Design review of the part built by this model. Coordinates are the model's own, in mm. Coordinates: 2 decimals unless noted, no trailing zeros. Order: outer loops, then holes, each group sorted by start corner. A loop starts at its lowest first (then second) coordinate and runs counter-clockwise, first axis right, second up. Notation, with made-up numbers: (48, 45) -> (87, 45) arc R26 ccw to (87, 74) -> close; hole circle Ø11 at (-32, 50). An arc over 180 degrees is marked (long way). Write item = value, one per line.
```python
from build123d import *

# Parameters (mm, degrees)
F0_W     = 58.954738
F0_H     = 37.899476
F1_DEPTH = 25.4
F2_R     = 5.08
F3_SIZE  = 5.08


with BuildPart() as f1:
    # F0 (on Front) → F1 (new body)
    with BuildSketch(Plane.XZ):
        Rectangle(F0_W, F0_H)
    extrude(amount=F1_DEPTH)

    # F2
    f2_edges = [f1.edges().sort_by_distance(p)[0] for p in [
        (0, -25.4, 18.949738),
        (0, -25.4, -18.949738),
    ]]
    fillet(f2_edges, radius=F2_R)

    # F3
    f3_edges = [f1.edges().sort_by_distance(p)[0] for p in [
        (0, 0, -18.949738),
        (0, 0, 18.949738),
    ]]
    chamfer(f3_edges, length=F3_SIZE)


solid = f1.part
```
(1) We need section C-C (y = -23). Write out the cut boundary in (x, z).
Report:
outline = (-29.48, -18.19) -> (29.48, -18.19) -> (29.48, 18.19) -> (-29.48, 18.19) -> close
(2) For L1, parallel to Z at x = -11.5, y = -3; L2, parallel to Z at x = -18.5, y = -3.25; L3, parallel to Y at x = -7, z = 16, list the stretches that pass through material, from the lowest coordinate up.
Report:
L1 = -16.87 to 16.87
L2 = -17.12 to 17.12
L3 = -24.93 to -2.13
(3) We need section A-A (x = 21). Write out the cut boundary in (y, z), and give its area (3 significant figures).
Report:
outline = (-25.4, -13.87) arc R5.08 ccw to (-20.32, -18.95) -> (-5.08, -18.95) -> (0, -13.87) -> (0, 13.87) -> (-5.08, 18.95) -> (-20.32, 18.95) arc R5.08 ccw to (-25.4, 13.87) -> close
area = 926 mm²
(4) We need section B-B (z = -16). Write out the cut boundary in (x, y).
Report:
outline = (-29.48, -24.93) -> (29.48, -24.93) -> (29.48, -2.13) -> (-29.48, -2.13) -> close
